```python
from build123d import *

# Parameters (mm, degrees)
SKETCH1_R           = 30
BOSS_EXTRUDE1_DEPTH = 20
SKETCH2_R           = 6.6
CUT_EXTRUDE1_DEPTH  = 10
SKETCH3_R           = 2
CUT_EXTRUDE2_DEPTH  = 35
CIRPATTERN1_COUNT   = 6
SKETCH6_R           = 1.75
CUT_EXTRUDE4_DEPTH  = 45
CIRPATTERN3_COUNT   = 4


with BuildPart() as part:
    # Sketch1 → Boss-Extrude1 (new body)
    with BuildSketch(Plane(origin=(0, 0, 0), x_dir=(1, 0, 0), z_dir=(0, 1, 0))):
        with Locations(Location((0, 0, 0), (0, 0, 270))):
            Circle(SKETCH1_R)
    extrude(amount=BOSS_EXTRUDE1_DEPTH)

    # Sketch2 → Cut-Extrude1 (cut)
    with BuildSketch(Plane(origin=(0, 20, 0), x_dir=(1, 0, 0), z_dir=(0, 1, 0))):
        with Locations(Location((0, 20, 0), (0, 0, 270))):
            Circle(SKETCH2_R)
    cut_extrude1 = extrude(amount=-CUT_EXTRUDE1_DEPTH, mode=Mode.SUBTRACT)

    # Sketch3 → Cut-Extrude2 (cut)
    with BuildSketch(Plane(origin=(0, 10, 0), x_dir=(1, 0, 0), z_dir=(0, 1, 0))):
        with Locations(Location((0, 20, 0), (0, 0, 270))):
            Circle(SKETCH3_R)
    cut_extrude2 = extrude(amount=-CUT_EXTRUDE2_DEPTH, mode=Mode.SUBTRACT)

    # CirPattern1: Cut-Extrude1, Cut-Extrude2 ×6 about axis
    cirpattern1_axis = Axis((0, 0, 0), (0, 1, 0))
    add([cut_extrude1.rotate(cirpattern1_axis, i * 360 / CIRPATTERN1_COUNT) for i in range(1, CIRPATTERN1_COUNT)], mode=Mode.SUBTRACT)
    add([cut_extrude2.rotate(cirpattern1_axis, i * 360 / CIRPATTERN1_COUNT) for i in range(1, CIRPATTERN1_COUNT)], mode=Mode.SUBTRACT)

    # Sketch6 → Cut-Extrude4 (cut)
    with BuildSketch(Plane(origin=(0, 20, 0), x_dir=(1, 0, 0), z_dir=(0, 1, 0))):
        with Locations(Location((4.5, 0, 0), (0, 0, 270))):
            Circle(SKETCH6_R)
    cut_extrude4 = extrude(amount=-CUT_EXTRUDE4_DEPTH, mode=Mode.SUBTRACT)

    # CirPattern3: Cut-Extrude4 ×4 about axis
    cirpattern3_axis = Axis((0, 0, 0), (0, 1, 0))
    for i in range(1, CIRPATTERN3_COUNT):
        add(cut_extrude4.rotate(cirpattern3_axis, i * 360 / CIRPATTERN3_COUNT), mode=Mode.SUBTRACT)

    # Sketch7 → Cut-Revolve1 (revolve, cut)
    with BuildSketch(Plane.XY, mode=Mode.PRIVATE) as cut_revolve1_sk:
        Polygon((-25, 0), (-25, 5), (-30, 10), (-30, 0), align=None)
    revolve(cut_revolve1_sk.sketch.rotate(Axis((0, 0, 0), (0, 1, 0)), 270), axis=Axis((0, 0, 0), (0, 1, 0)), mode=Mode.SUBTRACT)


solid = part.part
```
Check sheet for the modelled part. Datum: model origin and axes. Units: mm. A direction names the side the tool comes from. Give positions to 0.01 mm unless a question says otherwise; leave off trailing zeros. Write each loop counter-clockwise with the first axis right and the second up, starting at its lowest first coordinate (ties: lowest second). Pieces come first, ordered by that corner, then holes.
Item 1: Gauge pin test, flat ends, axial feed: pin 1 (21 mm diameter, centred on x = 0, z = 20, fed in from +Y); pin 2 (1 mm diameter, centred on y = 6, z = 11.5, fed in from -X); pin 3 (4 mm diameter, centred on y = 8.5, z = 23.5, fed in from +X); pin 4 (4 mm diameter, centred on x = 0.5, z = -23, fed in from +Y). Record the tip position at first contact, or that the pin passes through.
Item 2: Cross-section at A-A (z = 0). Enter the section's corners in (x, y).
Item 3: Scan lines: L1, parallel to X at y = 4.5, z = 0; L2, parallel to Z at x = -4.5, y = 15.25; L3, parallel to Z at x = -18, y = 17. Record each from-to range of solid material in increasing order.
Item 4: Draft check along X on faces 3 (the face through (-2.79, 10.14, 0.38)), 4 (the face through (15, 10, 11)), 5 (the face through (-7.509, 2.535, -23.846)). Enter one of: released by +X, released by -X, zero draft, split by the parting line, or undercut.
Item 5: Access from +Z, -Z, +X, -X, +Y, -Y to the whole of each face (thin tool, end or side, straight path). Record for faces 1 (the face through (-1, 10, -22)), 2 (the face through (-1.2, 5.1, -21.6)).
Item 6: Cross-section at B-B (x = 0). Count the separate pieces of the cut face and the enclosed holes in it, and give its area (3 significant figures).
Report:
1. pin 1: stops at y = 20
1. pin 2: stops at x = -23.92
1. pin 3: stops at x = 20.2
1. pin 4: stops at y = 10
2. outline: (-30, 10) - (-25, 5) - (-25, 0) - (-6.25, 0) - (-6.25, 20) - (-30, 20) - close; (-2.75, 0) - (2.75, 0) - (2.75, 20) - (-2.75, 20) - close; (6.25, 0) - (25, 0) - (25, 5) - (30, 10) - (30, 20) - (6.25, 20) - close
3. L1: x = -25 to -6.25, -2.75 to 2.75, 6.25 to 25
3. L2: z = -29.66 to -24.83, -15.17 to -1.75, 1.75 to 15.17, 24.83 to 29.66
3. L3: z = -24 to -16.56, -3.44 to 3.44, 16.56 to 24
4. face 3: undercut
4. face 4: undercut
4. face 5: split by the parting line
5. face 1: +Y
5. face 2: +Y, -Y
6. separate pieces: 5
6. enclosed holes: 0
6. area: 641 mm2
